Study the drawing (mm; zero at the part's minimum x, y, z) and answer. A direction names the side the tool comes from. Give positions to 0.01 mm unless a question says otherwise; leave off trailing zeros. Order: outer loops, then holes, each group sorted by start corner. A loop starts at its lowest first (then second) coordinate and runs counter-clockwise, first axis right, second up.
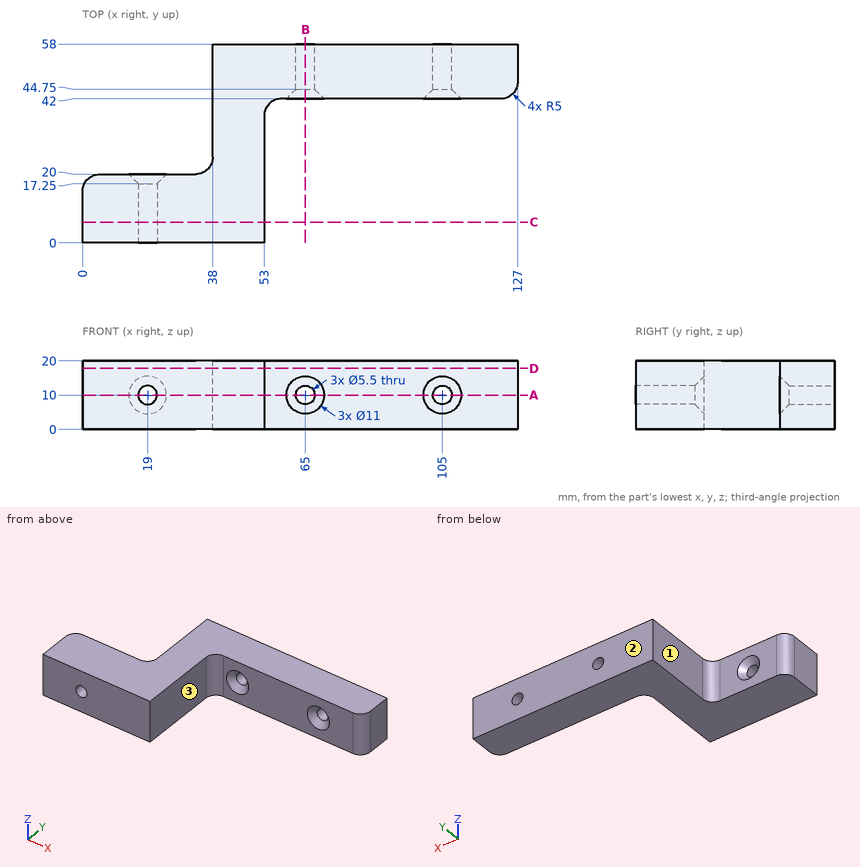
1) A tool of negligible diameter and unlimited length cuts with its end or side. For the marked faces 1, 2 and 3, from which of +Z, -Z, +X, -X, +Y, -Y can it reach the whole face along a straight path? Write none if from no direction.
Geometry says:
face 1: +Z, -Z, -X, +Y
face 2: +Z, -Z, +X, -X, +Y
face 3: +Z, -Z, +X, -Y
2) Given P1, Ø12, axis at y = 48, z = 6, coming from the -X side; P2, Ø2, axis at y = 42, z = 7, coming from the +X side; P3, Ø7, axis at x = 19, z = 10, coming from the +Y side, each flat-ended and moving along its own axis, determine where each tip first touches the part or whether it passes through.
Geometry says:
P1: stops at x = 38
P2: stops at x = 125
P3: stops at y = 18
3) Find section B-B (x = 65). Write down the section's boundary in (y, z), then the cut area to 3 significant figures.
Geometry says:
outline: (42, 0) - (58, 0) - (58, 7.25) - (44.75, 7.25) - (42, 4.5) - close; (42, 15.5) - (44.75, 12.75) - (58, 12.75) - (58, 20) - (42, 20) - close
area: 224 mm2
4) Find section D-D (z = 17.75). Write down the section's boundary in (x, y).
Geometry says:
outline: (0, 0) - (53, 0) - (53, 37) arc R5 cw to (58, 42) - (122, 42) arc R5 ccw to (127, 47) - (127, 58) - (38, 58) - (38, 25) arc R5 cw to (33, 20) - (5, 20) arc R5 ccw to (0, 15) - close
5) Find section C-C (y = 6). Write down the section's boundary in (x, z).
Geometry says:
outline: (0, 0) - (53, 0) - (53, 20) - (0, 20) - close; hole circle Ø5.5 at (19, 10)
6) Find section A-A (z = 10). Count the separate pieces of the cut face and the enclosed holes in it, then the cut area to 3 significant figures.
Geometry says:
separate pieces: 4
enclosed holes: 0
area: 2,510 mm2
7) Straight lines are drawn through the part: probe 1 along X at (y, z) = (53.25, 10); probe 2 along X at (y, z) = (13.5, 10); probe 3 along Z at (x, y) = (65, 48.25). For each, find the intervals that lie inside material, in ascending order.
Geometry says:
probe 1: x = 38 to 62.25, 67.75 to 102.25, 107.75 to 127
probe 2: x = 0 to 16.25, 21.75 to 53
probe 3: z = 0 to 7.25, 12.75 to 20
